from build123d import *

# Parameters (mm, degrees)
F1_DEPTH  = 7.9375
F2_W      = 3.96875
F2_H      = 7.9375
F3_DEPTH  = 15.875
F4_R      = 3.96874
F5_W      = 1.56845
F5_H      = 1.6891
F5_W_2    = 1.6891
F5_H_2    = 1.56845
F5_R      = 2.54
F6_DEPTH  = 23.8125
F8_DEPTH  = 3.96875
F10_DEPTH = 3.96875


# Not quite as in the source:
# - a fillet or chamfer is up to 0.001 mm smaller than in the source, because OpenCascade refuses the exact size


with BuildPart() as f1:
    # F0 (on Top) → F1 (new body)
    with BuildSketch(Plane.XY):
        Polygon((0, 82.7019174), (0, 0), (7.9375, 0), (7.9375, 31.75), (15.875, 31.75), (15.875, 0), (23.8125, 0), (23.8125, 82.7019174), (15.875, 82.7019174), (15.875, 98.5769174), (7.9375, 98.5769174), (7.9375, 82.7019174), align=None)
    extrude(amount=F1_DEPTH)

    # F2 (on face) → F3 (join)
    with BuildSketch(Plane(origin=(0, 0, 0), x_dir=(1, 0, 0), z_dir=(0, 0, -1))):
        with Locations((21.828125, -47.5457774)):
            Rectangle(F2_W, F2_H)
        with Locations((1.984375, -47.5457774)):
            Rectangle(F2_W, F2_H)
    extrude(amount=F3_DEPTH)

    # F4 (radius 3.96875 in the source; OpenCascade refuses exactly that, so slightly less here)
    f4_edges = [f1.edges().sort_by_distance(p)[0] for p in [
        (19.84375, 82.701917, 0),
        (19.84375, 82.701917, 7.9375),
        (11.90625, 98.576917, 0),
        (11.90625, 98.576917, 7.9375),
        (3.96875, 82.701917, 0),
        (3.96875, 82.701917, 7.9375),
        (1.984375, 51.514527, -15.875),
        (1.984375, 43.577027, -15.875),
        (21.828125, 51.514527, -15.875),
        (21.828125, 43.577027, -15.875),
        (3.96875, 0, 0),
        (3.96875, 0, 7.9375),
        (19.84375, 0, 7.9375),
        (19.84375, 0, 0),
        (11.90625, 31.75, 7.9375),
        (11.90625, 31.75, 0),
    ]]
    fillet(f4_edges, radius=F4_R)

    # F5 (on face) → F6 (cut, through all)
    with BuildSketch(Plane(origin=(0, 0, 0), x_dir=(0, -1, 0), z_dir=(-1, 0, 0))):
        with Locations((-2.339975, 3.96875)):
            Rectangle(F5_W, F5_H)
        with Locations((-3.96875, 2.339975)):
            Rectangle(F5_W_2, F5_H_2)
        with Locations((-3.96875, 3.96875)):
            Rectangle(F5_W_2, F5_H)
        with Locations((-5.597525, 3.96875)):
            Rectangle(F5_W, F5_H)
        with Locations((-3.96875, 5.597525)):
            Rectangle(F5_W_2, F5_H_2)
        with Locations((-47.5457774, -10.277475)):
            Rectangle(F5_W_2, F5_H_2)
        with Locations((-47.5457774, -11.90625)):
            Rectangle(F5_W_2, F5_H)
        with Locations((-49.1745524, -11.90625)):
            Rectangle(F5_W, F5_H)
        with Locations((-45.9170024, -11.90625)):
            Rectangle(F5_W, F5_H)
        with Locations((-47.5457774, -13.535025)):
            Rectangle(F5_W_2, F5_H_2)
        with Locations((-19.84375, 2.339975)):
            Rectangle(F5_W_2, F5_H_2)
        with Locations((-21.472525, 3.96875)):
            Rectangle(F5_W, F5_H)
        with Locations((-19.84375, 3.96875)):
            Rectangle(F5_W_2, F5_H)
        with Locations((-18.214975, 3.96875)):
            Rectangle(F5_W, F5_H)
        with Locations((-19.84375, 5.597525)):
            Rectangle(F5_W_2, F5_H_2)
        with Locations((-94.6081674, 3.96875)):
            Circle(F5_R)
    extrude(amount=-F6_DEPTH, mode=Mode.SUBTRACT)

    # F7 (on face) → F8 (join, through all)
    with BuildSketch(Plane(origin=(0, 0, 0), x_dir=(0, -1, 0), z_dir=(-1, 0, 0))):
        with BuildLine():
            Line((-65.0646874757, 0), (-50.3521074378, -14.7125800378))
            ThreePointArc((-50.3521074378, -14.7125800378), (-51.2124242947, -13.4250248722), (-51.5145274, -11.90625))
            Line((-51.5145274, -11.90625), (-51.5145274, 0))
            Line((-51.5145274, 0), (-65.0646874757, 0))
        make_face()
    extrude(amount=-F8_DEPTH)

    # F9 (on face) → F10 (join, through all)
    with BuildSketch(Plane.YZ.offset(23.8125)):
        with BuildLine():
            ThreePointArc((51.5145274, -11.90625), (51.2124242947, -13.4250248722), (50.3521074378, -14.7125800378))
            Line((50.3521074378, -14.7125800378), (65.0646874757, 0))
            Line((65.0646874757, 0), (51.5145274, 0))
            Line((51.5145274, 0), (51.5145274, -11.90625))
        make_face()
    extrude(amount=-F10_DEPTH)


solid = f1.part
Model file for the job. Use its own axes, mm. A direction names the side the tool comes from. Give positions to 0.01 mm unless a question says otherwise; leave off trailing zeros. Write each loop counter-clockwise with the first axis right and the second up, starting at its lowest first coordinate (ties: lowest second). Pieces come first, ordered by that corner, then holes. Notation, with made-up numbers: (-36.75, 75) - (-31.75, 75) arc R20 ccw to (-31.75, 105) - close; hole circle Ø3 at (67, 31). An arc over 180 degrees is marked (long way). Answer as CSV lines item,"result".
1. Band-saw the part on C-C (z = -4.25). Write the cut outline in (x, y), and give its area (3 significant figures).
Responses:
outline,"(0, 43.58) - (3.97, 43.58) - (3.97, 60.81) - (0, 60.81) - close; (19.84, 43.58) - (23.81, 43.58) - (23.81, 60.81) - (19.84, 60.81) - close"
area,"137 mm2"
2. 3-axis set-ups, long thin cutter, end or side, ignore diameter. For faces 1 (the face through (2, 43.577, -6)), 2 (the face through (4, 18, 3.124)): which of +Z, -Z, +X, -X, +Y, -Y reach the whole face in a straight line?
Responses:
face 1,"-Z, +X, -X, -Y"
face 2,"+X, -X"
3. Band-saw the part on D-D (y = 55). Write the cut outline in (x, z), and give its area (3 significant figures).
Responses:
outline,"(0, -10.06) - (3.97, -10.06) - (3.97, 0) - (19.84, 0) - (19.84, -10.06) - (23.81, -10.06) - (23.81, 7.94) - (0, 7.94) - close"
area,"269 mm2"
4. Band-saw the part on B-B (y = 10). Write the cut outline in (x, z) (1 decimal), and give its area (3 significant figures).
Responses:
outline,"(0, 0) - (7.9, 0) - (7.9, 7.9) - (0, 7.9) - close; (15.9, 0) - (23.8, 0) - (23.8, 7.9) - (15.9, 7.9) - close"
area,"126 mm2"
5. Two-plate mould, pull along Y, no slides. Class faces 3 (the face through (3.969, 52, -6)), 4 (the face through (4, 20, 6.382)), 5 (the face through (1.957, 57.813, -7.251)): +Y half, -Y half, draft (parallel to the pull), parting line (faces both ways), or undercut.
Responses:
face 3,"draft"
face 4,"undercut"
face 5,"+Y half"
6. Pin check, flat tips, straight feed: pin 1 (8 mm diameter, centred on x = 15, y = 62, fed in from -Z); pin 2 (0.5 mm diameter, centred on x = 2.5, z = -12, fed in from -Y); pin 3 (1 mm diameter, centred on x = 3.5, y = 63, fed in from -Z); pin 4 (5 mm diameter, centred on y = 73, z = 1, fed in from -X). Stop position of each tip, or through.
Responses:
pin 1,"stops at z = 0"
pin 2,"stops at y = 43.58"
pin 3,"stops at z = -2.56"
pin 4,"stops at x = 0"
7. Drill centre lines: L1, parallel to X at y = 49, z = -13; L2, parallel to Y at x = 3.5, z = 2; L3, parallel to X at y = 21.5, z = 2 (1 decimal). Where is each one in solid material? Low to high. Write a range as [from, to].
Responses:
L1,"x = [0, 3.97], [19.84, 23.81]"
L2,"y = [0.52, 3.12], [4.81, 19], [20.69, 82.18]"
L3,"x = [0, 7.9], [15.9, 23.8]"
